from build123d import *

# Parameters (mm, degrees)
CUT_EXTRUDE1_DEPTH      = 348.634865915
CUT_EXTRUDE1_DEPTH_BACK = 348.634865915
SKETCH2_R               = 8
CUT_EXTRUDE2_DEPTH      = 357.16007637
CUT_EXTRUDE2_DEPTH_BACK = 357.16007637


with BuildPart() as part:
    # Sketch1 → Revolve1 (revolve)
    with BuildSketch(Plane.XY, mode=Mode.PRIVATE) as revolve1_sk:
        with BuildLine():
            Line((27.5, 0), (65, 0))
            ThreePointArc((65, 0), (72.071067812, 2.928932188), (75, 10))
            Line((75, 10), (75, 35))
            ThreePointArc((75, 35), (85.251262658, 59.748737342), (110, 70))
            Line((110, 70), (175, 70))
            Line((175, 70), (175, 105))
            Line((175, 105), (225, 105))
            Line((225, 105), (225, 130))
            ThreePointArc((225, 130), (222.071067812, 137.071067812), (215, 140))
            Line((215, 140), (110, 140))
            Line((110, 140), (77.808672972, 112.407433976))
            ThreePointArc((77.808672972, 112.407433976), (74.770221715, 110.621149851), (71.300759238, 110))
            Line((71.300759238, 110), (49.049875621, 110))
            ThreePointArc((49.049875621, 110), (42.339822414, 112.585474664), (39.099503719, 119.00496281))
            Line((39.099503719, 119.00496281), (35, 160))
            Line((35, 160), (27.5, 160))
            Line((27.5, 160), (27.5, 0))
        make_face()
    revolve(revolve1_sk.sketch.rotate(Axis((0, 0, 0), (0, 1, 0)), 90), axis=Axis((0, 0, 0), (0, 1, 0)))

    # Sketch2 → Cut-Extrude1 (cut, two sides: drawn at the far end of the back side and taken through both)
    with BuildSketch(Plane(origin=(0, 140, 0), x_dir=(1, 0, 0), z_dir=(0, 1, 0)).offset(-CUT_EXTRUDE1_DEPTH_BACK)):
        with Locations(Location((200, 0, 0), (0, 0, 270))):
            Circle(SKETCH2_R)
        with Locations(Location((100, -173.205080757, 0), (0, 0, 270))):
            Circle(SKETCH2_R)
        with Locations(Location((-100, -173.205080757, 0), (0, 0, 270))):
            Circle(SKETCH2_R)
        with Locations(Location((-200, 0, 0), (0, 0, 270))):
            Circle(SKETCH2_R)
        with Locations(Location((-100, 173.205080757, 0), (0, 0, 270))):
            Circle(SKETCH2_R)
        with Locations(Location((100, 173.205080757, 0), (0, 0, 270))):
            Circle(SKETCH2_R)
    extrude(amount=CUT_EXTRUDE1_DEPTH + CUT_EXTRUDE1_DEPTH_BACK, mode=Mode.SUBTRACT)

    # Sketch3 → Cut-Extrude2 (cut, two sides: drawn at the far end of the back side and taken through both)
    with BuildSketch(Plane(origin=(0, 160, 0), x_dir=(1, 0, 0), z_dir=(0, 1, 0)).offset(-CUT_EXTRUDE2_DEPTH_BACK)):
        with BuildLine():
            Line((-8, 26.310644234), (-8, 31.8))
            Line((-8, 31.8), (8, 31.8))
            Line((8, 31.8), (8, 26.310644234))
            ThreePointArc((8, 26.310644234), (0, 27.5), (-8, 26.310644234))
        make_face()
    extrude(amount=CUT_EXTRUDE2_DEPTH + CUT_EXTRUDE2_DEPTH_BACK, mode=Mode.SUBTRACT)


solid = part.part
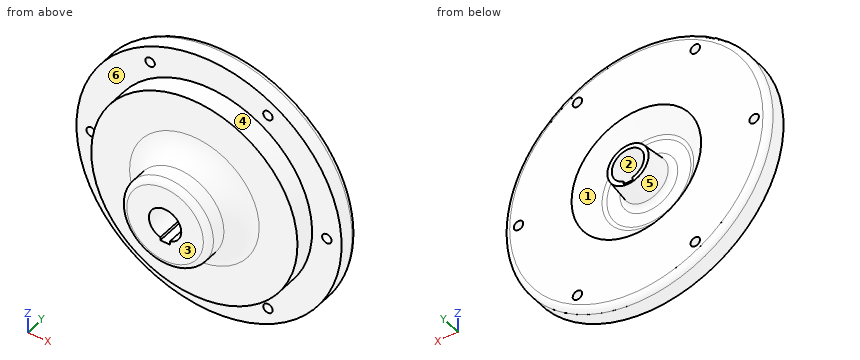
Could you check a few things on this model? Use its own coordinates, in mm. Face numbers are marked on the shaded views. A direction names the side the tool comes from. Round coordinates to 2 decimals unless told otherwise and drop trailing zeros. Loops run counter-clockwise (first coordinate to the right, second up) from the corner with the lowest first, then second, coordinate; pieces in that order, holes last. Notation, with made-up numbers: (15.25, 42.5) -> (27.25, 42.5) arc R17 ccw to (27.25, 47.5) -> close; hole circle Ø7 at (72, 58). An arc over 180 degrees is marked (long way). Use CSV: the item, a comma, the result in double quotes.
(1) Will these pins go through, and if not, where does the flat tip stop? pin 1 Ø5 at (x, y) = (0, 102) entering from +Z; pin 2 Ø10 at (x, y) = (110, 111.5) entering from +Z; pin 3 Ø4 at (x, z) = (-104, 13.5) entering from +Y.
Return value:
pin 1,"stops at z = 175"
pin 2,"stops at z = 199"
pin 3,"stops at y = 137.32"
(2) Suppose I cut it at C-C on z = 0. Give the number of separate pieces and of enclosed holes in the cut face, plus the area to 3 significant figures.
Return value:
separate pieces,"4"
enclosed holes,"0"
area,"27,300 mm²"
(3) Suppose I cut it at B-B on y = 96. Write out the boundary of the cut face in (x, z), plus the area to 3 significant figures.
Return value:
outline,"circle Ø350 at (0, 0); hole (-8, -31.8) -> (8, -31.8) -> (8, -26.31) arc R27.5 ccw (long way) to (-8, -26.31) -> close"
area,"93,800 mm²"
(4) If we mould it in two halves opening along X, with no side actions, what happens to the marked faces 1, 2, 3 and 4? For each: +X half, -X half, draft (parallel to the pull), parting line (faces both ways), or undercut.
Return value:
face 1,"undercut"
face 2,"undercut"
face 3,"draft"
face 4,"parting line"
(5) For the marked faces 5 and 6, which set-ups out of +Z, -Z, +X, -X, +Y, -Y let a thin tool reach every point of the face, with its end or its side?
Return value:
face 5,"+Y"
face 6,"-Y"
(6) If I drill on probe 1 along X at (y, z) = (113.5, 0); probe 2 along Z at (x, y) = (-100, 124); probe 3 along X at (y, z) = (126, 0), over which ranges is the centre line in solid material (lowest first)? Write a range as [from, to].
Return value:
probe 1,"x = [-225, -208], [-192, -79.08], [-41.45, -27.5], [27.5, 41.45], [79.08, 192], [208, 225]"
probe 2,"z = [-201.56, -181.21], [-165.21, 165.21], [181.21, 201.56]"
probe 3,"x = [-225, -208], [-192, -93.67], [-38.4, -27.5], [27.5, 38.4], [93.67, 192], [208, 225]"
